Model file for the job. Use its own axes, mm. A direction names the side the tool comes from. Give positions to 0.01 mm unless a question says otherwise; leave off trailing zeros. Loops run counter-clockwise (first coordinate to the right, second up) from the corner with the lowest first, then second, coordinate; pieces in that order, holes last. Notation, with made-up numbers: M -24.75,59.25 L 23.25,59.25 A19 ccw 23.25,70.25 Z; hole C 70.25,70.25 d4. An arc over 180 degrees is marked long. Answer in a Markdown table with one row per item.
```python
from build123d import *

# Parameters (mm, degrees)
SALIENTE_EXTRUIR1_DEPTH = 60
CROQUIS2_R              = 3.5
CORTAR_EXTRUIR1_DEPTH   = 60
REDONDEO1_R             = 1
CHAFL_N1_SIZE           = 1


with BuildPart() as part:
    # Croquis1 → Saliente-Extruir1 (new body)
    with BuildSketch(Plane.XY):
        Polygon((3.538389259, 50.854615385), (3.538389259, 25.854615385), (-13.791610741, 25.854615385), (-13.791610741, -4.145384615), (-10.621610741, -4.145384615), (-10.621610741, 22.684615385), (6.708389259, 22.684615385), (6.708389259, 50.854615385), align=None)
    extrude(amount=SALIENTE_EXTRUIR1_DEPTH)

    # Croquis2 → Cortar-Extruir1 (cut)
    with BuildSketch(Plane(origin=(6.708389259, 0, 0), x_dir=(0, 0, -1), z_dir=(1, 0, 0))):
        with Locations(Location((-53, 44.854615385, 0), (0, 0, 90))):
            Circle(CROQUIS2_R)
        with Locations(Location((-53, 31.854615385, 0), (0, 0, 90))):
            Circle(CROQUIS2_R)
        with Locations(Location((-7, 44.854615385, 0), (0, 0, 90))):
            Circle(CROQUIS2_R)
        with Locations(Location((-7, 31.854615385, 0), (0, 0, 90))):
            Circle(CROQUIS2_R)
    extrude(amount=-CORTAR_EXTRUIR1_DEPTH, mode=Mode.SUBTRACT)

    # Redondeo1
    redondeo1_edges = [part.edges().sort_by_distance(p)[0] for p in [
        (-10.621610741, 22.684615385, 30),
        (3.538389259, 25.854615385, 30),
    ]]
    fillet(redondeo1_edges, radius=REDONDEO1_R)

    # Chaflán1
    chafl_n1_edges = [part.edges().sort_by_distance(p)[0] for p in [
        (-13.791610741, 10.854615385, 0),
        (3.538389259, 38.854615385, 0),
        (5.123389259, 50.854615385, 0),
        (-10.621610741, -4.145384615, 30),
        (-13.791610741, -4.145384615, 30),
        (-13.791610741, 25.854615385, 30),
        (3.538389259, 50.854615385, 30),
        (-13.791610741, 10.854615385, 60),
        (-10.621610741, 8.769615385, 60),
        (6.708389259, 36.769615385, 60),
        (-1.456610741, 22.684615385, 0),
        (-1.456610741, 22.684615385, 60),
        (-5.626610741, 25.854615385, 0),
        (-5.626610741, 25.854615385, 60),
        (-10.328717522, 22.391722166, 0),
        (-10.328717522, 22.391722166, 60),
        (3.24549604, 26.147508603, 0),
        (3.24549604, 26.147508603, 60),
        (6.708389259, 36.769615385, 0),
        (3.538389259, 38.854615385, 60),
        (-10.621610741, 8.769615385, 0),
        (-12.206610741, -4.145384615, 0),
    ]]
    chamfer(chafl_n1_edges, length=CHAFL_N1_SIZE)


solid = part.part
```
(1) Saw through at C-C, the plane x = 1. Give the cut face in (y, z).
Established:
| item | result |
|---|---|
| outline | M 22.68,1 L 23.68,0 L 24.85,0 L 25.85,1 L 25.85,59 L 24.85,60 L 23.68,60 L 22.68,59 Z |
(2) Saw through at B-B, the plane y = 44. Give the cut face in (x, z), and give its area (3 significant figures).
Established:
| item | result |
|---|---|
| outline | M 3.54,1 L 4.54,0 L 5.71,0 L 6.71,1 L 6.71,3.61 L 3.54,3.61 Z; M 3.54,10.39 L 6.71,10.39 L 6.71,49.61 L 3.54,49.61 Z; M 3.54,56.39 L 6.71,56.39 L 6.71,59 L 5.71,60 L 4.54,60 L 3.54,59 Z |
| area | 145 mm2 |
(3) Saw through at A-A, the plane z = 7. Give the cut face in (x, y), and give its area (3 significant figures).
Established:
| item | result |
|---|---|
| outline | M -13.79,-3.15 L -12.79,-4.15 L -11.62,-4.15 L -10.62,-3.15 L -10.62,21.68 A1 cw -9.62,22.68 L 6.71,22.68 L 6.71,28.35 L 3.54,28.35 L 3.54,26.85 A1 cw 2.54,25.85 L -12.79,25.85 L -13.79,24.85 Z; M 3.54,35.35 L 6.71,35.35 L 6.71,41.35 L 3.54,41.35 Z; M 3.54,48.35 L 6.71,48.35 L 6.71,50.85 L 4.54,50.85 L 3.54,49.85 Z |
| area | 183 mm2 |
(4) Wall check: L1, parallel to Y at x = 4, z = 9; L2, parallel to Z at x = 6, y = 34; L3, parallel to Y at x = -3, z = 53.5. Give the ranges that are in metal, low to high.
Established:
| item | result |
|---|---|
| L1 | y = 22.68 to 28.98, 34.73 to 41.98, 47.73 to 50.32 |
| L2 | z = 0.29 to 4.23, 9.77 to 50.23, 55.77 to 59.71 |
| L3 | y = 22.68 to 25.85 |
(5) Mould opens along Y. For faces 1 (the conical face through (3.54, 25.88, 0.6)), 2 (the cylindrical face through (5.15, 48.09, 5.66)), 3 (the conical face through (-10.61, 22.65, 59.38)) say: pulls with the +Y half, pulls with the -Y half, needs draft (parallel to the pull), parting line crosses it, or undercut.
Established:
| item | result |
|---|---|
| face 1 | pulls with the +Y half |
| face 2 | undercut |
| face 3 | pulls with the -Y half |
(6) Flat gauge pins, fed straight in: P1, Ø4, axis at y = 31.85, z = 7, coming from the +X side; P2, Ø4, axis at x = 3, z = 9.5, coming from the -Y side; P3, Ø8, axis at y = 44.85, z = 7, coming from the -X side; P4, Ø12, axis at x = -7.5, y = 19, coming from the -Z side. Where does each tip first touch, or does it go through?
Established:
| item | result |
|---|---|
| P1 | passes through |
| P2 | stops at y = 22.68 |
| P3 | stops at x = 3.54 |
| P4 | stops at z = 0 |
(7) Saw through at D-D, the plane z = 23. Give the cut face in (x, y).
Established:
| item | result |
|---|---|
| outline | M -13.79,-3.15 L -12.79,-4.15 L -11.62,-4.15 L -10.62,-3.15 L -10.62,21.68 A1 cw -9.62,22.68 L 6.71,22.68 L 6.71,50.85 L 4.54,50.85 L 3.54,49.85 L 3.54,26.85 A1 cw 2.54,25.85 L -12.79,25.85 L -13.79,24.85 Z |
(8) Which spindle directions (+Z, -Z, +X, -X, +Y, -Y) get a long thin tool onto all of the face, cutting with end or side? Do faces 4 (the flat face through (6.708, 37, 30)), 5 (the flat face through (3.538, 39, 30)), 6 (the flat face through (-10.622, 9, 30)). Say none if no direction does.
Established:
| item | result |
|---|---|
| face 4 | +Z, -Z, +X, +Y, -Y |
| face 5 | +Z, -Z, -X, +Y |
| face 6 | +Z, -Z, +X, -Y |
